Here's how the part is built. I have some questions about the finished solid (model axes, mm). Face numbers are marked on the shaded views. A direction names the side the tool comes from. Coordinates: 2 decimals unless noted, no trailing zeros. Write each loop counter-clockwise with the first axis right and the second up, starting at its lowest first coordinate (ties: lowest second). Pieces come first, ordered by that corner, then holes. Notation, with made-up numbers: (39, 11) - (49, 11) arc R21 ccw to (49, 34) - close; hole circle Ø7 at (29.25, 82). An arc over 180 degrees is marked (long way). Answer in a Markdown table with one row per item. Add a question column.
Item 1: If I drill on probe 1 along Y at (x, z) = (-159.65, 102.5); probe 2 along Z at (x, y) = (-158, 177); probe 3 along Y at (x, z) = (-159, -102), over which ranges is the centre line in solid material (lowest first)? Write a range as from..to.
Item 2: We'd pull the mould along Z, two halves only. Please class the marked faces 6, 7 and 8: +Z half, -Z half, draft (parallel to the pull), parting line (faces both ways), or undercut.
Item 3: Which directions (+Z, -Z, +X, -X, +Y, -Y) give clear straight access to the entire face, cutting with the end or side of a thin tool? Please do the marked faces 1, 2, 3, 4 and 5.
Item 4: Imagine slicing it at B-B (z = 41.5). Please give me the cut outline in (x, y).
Item 5: I'm going to push flat-ended pins straight in: pin 1 (6.5 mm diameter, centred on y = 6, z = -86, fed in from -X); pin 2 (1 mm diameter, centred on x = 98, y = 65, fed in from -Z); pin 3 (10 mm diameter, centred on x = -37, y = 99, fed in from +Z); pin 4 (1.5 mm diameter, centred on x = -83.5, z = 106.5, fed in from -Y). Where does each tip first touch, or does it pass through?
Item 6: Imagine slicing it at A-A (x = -112.5). Please give me the cut outline in (y, z).
from build123d import *

# Parameters (mm, degrees)
BOSS_EXTRUDE1_DEPTH = 170
SKETCH3_W           = 20
SKETCH3_H           = 25
SKETCH3_R           = 5
SKETCH3_W_2         = 30
SKETCH3_H_2         = 30
BOSS_EXTRUDE2_DEPTH = 5
FILLET1_R           = 5
SKETCH5_R           = 3
CUT_EXTRUDE1_DEPTH  = 3
BOSS_EXTRUDE5_DEPTH = 15
CHAMFER1_SIZE       = 5
FILLET2_R           = 5
SKETCH15_R          = 3
CUT_EXTRUDE2_DEPTH  = 5
SKETCH16_R          = 3
CUT_EXTRUDE3_DEPTH  = 5
SKETCH18_W          = 20
SKETCH18_H          = 165
CUT_EXTRUDE9_DEPTH  = 5
SKETCH21_W          = 20
SKETCH21_H          = 165
CUT_EXTRUDE10_DEPTH = 5


with BuildPart() as part:
    # Sketch1 → Boss-Extrude1 (new body)
    with BuildSketch(Plane(origin=(0, 0, 0), x_dir=(1, 0, 0), z_dir=(0, 1, 0))):
        Polygon((162.5, 80), (162.5, -80), (152.5, -80), (147.5, -80), (132.5, -80), (132.5, -95), (132.5, -100), (132.5, -110), (-102.5, -110), (-102.5, -100), (-102.5, -85), (-112.5, -85), (-122.5, -85), (-122.5, -100), (-122.5, -110), (-162.5, -110), (-162.5, -100), (-162.5, -95), (-132.5, -95), (-132.5, -85), (-132.5, -75), (-93.003639463, -75), (-93.003639463, -100), (122.5, -100), (122.5, -70), (152.5, -70), (152.5, 70), (122.5, 70), (122.5, 100), (-93.003639463, 100), (-93.003639463, 75), (-132.5, 75), (-132.5, 85), (-132.5, 95), (-162.5, 95), (-162.5, 100), (-162.5, 110), (-122.5, 110), (-122.5, 100), (-122.5, 85), (-112.5, 85), (-102.5, 85), (-102.5, 100), (-102.5, 110), (132.5, 110), (132.5, 100), (132.5, 95), (132.5, 80), (147.5, 80), (152.5, 80), align=None)
    extrude(amount=BOSS_EXTRUDE1_DEPTH)

    # Sketch3 → Boss-Extrude2 (add)
    # profile 1 of 4: a face of its own
    with BuildSketch(Plane(origin=(0, 0, 0), x_dir=(1, 0, 0), z_dir=(0, 1, 0))):
        with Locations((-112.5, -97.5)):
            Rectangle(SKETCH3_W, SKETCH3_H)
        with Locations(Location((-112.5, -95, 0), (0, 0, 270))):
            Circle(SKETCH3_R, mode=Mode.SUBTRACT)
    # profile 2 of 4: a face of its own
    with BuildSketch(Plane(origin=(0, 0, 0), x_dir=(1, 0, 0), z_dir=(0, 1, 0))):
        with Locations((147.5, -95)):
            Rectangle(SKETCH3_W_2, SKETCH3_H_2)
        with Locations(Location((147.5, -95, 0), (0, 0, 270))):
            Circle(SKETCH3_R, mode=Mode.SUBTRACT)
    # profile 3 of 4: a face of its own
    with BuildSketch(Plane(origin=(0, 0, 0), x_dir=(1, 0, 0), z_dir=(0, 1, 0))):
        with Locations((-112.5, 97.5)):
            Rectangle(SKETCH3_W, SKETCH3_H)
        with Locations(Location((-112.5, 95, 0), (0, 0, 90))):
            Circle(SKETCH3_R, mode=Mode.SUBTRACT)
    # profile 4 of 4: a face of its own
    with BuildSketch(Plane(origin=(0, 0, 0), x_dir=(1, 0, 0), z_dir=(0, 1, 0))):
        with Locations((147.5, 95)):
            Rectangle(SKETCH3_W_2, SKETCH3_H_2)
        with Locations(Location((147.5, 95, 0), (0, 0, 270))):
            Circle(SKETCH3_R, mode=Mode.SUBTRACT)
    extrude(amount=BOSS_EXTRUDE2_DEPTH)

    # Fillet1
    fillet1_edges = [part.edges().sort_by_distance(p)[0] for p in [
        (-122.5, 87.5, 85),
        (-102.5, 87.5, 85),
        (132.5, 87.5, 80),
        (132.5, 87.5, -80),
        (-102.5, 87.5, -85),
        (-122.5, 87.5, -85),
    ]]
    fillet(fillet1_edges, radius=FILLET1_R)

    # Sketch5 → Cut-Extrude1 (cut)
    with BuildSketch(Plane.ZY.offset(132.5)):
        with Locations((-85, 5)):
            Circle(SKETCH5_R)
        with Locations(Location((85, 5, 0), (0, 0, 180))):
            Circle(SKETCH5_R)
        with Locations((-85, 165)):
            Circle(SKETCH5_R)
        with Locations(Location((85, 165, 0), (0, 0, 180))):
            Circle(SKETCH5_R)
    extrude(amount=-CUT_EXTRUDE1_DEPTH, mode=Mode.SUBTRACT)

    # Sketch10 → Boss-Extrude5 (add)
    with BuildSketch(Plane(origin=(0, 170, 0), x_dir=(1, 0, 0), z_dir=(0, 1, 0))):
        Polygon((-162.5, 95), (-162.5, -95), (-162.5, -100), (-162.5, -110), (-122.5, -110), (-122.5, -100), (-122.5, -85), (-112.5, -85), (-102.5, -85), (-102.5, -100), (-102.5, -110), (132.5, -110), (132.5, -100), (132.5, -95), (132.5, -80), (147.5, -80), (152.5, -80), (162.5, -80), (162.5, 80), (152.5, 80), (147.5, 80), (132.5, 80), (132.5, 95), (132.5, 100), (132.5, 110), (-102.5, 110), (-102.5, 100), (-102.5, 85), (-112.5, 85), (-122.5, 85), (-122.5, 100), (-122.5, 110), (-162.5, 110), (-162.5, 100), align=None)
    extrude(amount=BOSS_EXTRUDE5_DEPTH)

    # Chamfer1
    chamfer1_edges = [part.edges().sort_by_distance(p)[0] for p in [
        (147.5, 185, -80),
        (15, 185, -110),
        (-142.5, 185, -110),
        (-142.5, 185, 110),
        (15, 185, 110),
        (147.5, 185, 80),
    ]]
    chamfer(chamfer1_edges, length=CHAMFER1_SIZE)

    # Fillet2
    fillet2_edges = [part.edges().sort_by_distance(p)[0] for p in [
        (-122.5, 177.5, -85),
        (-102.5, 177.5, -85),
        (132.5, 175, -80),
        (132.5, 175, 80),
        (-102.5, 177.5, 85),
        (-122.5, 177.5, 85),
    ]]
    fillet(fillet2_edges, radius=FILLET2_R)

    # Sketch15 → Cut-Extrude2 (cut)
    with BuildSketch(Plane.XZ):
        with Locations(Location((67.5, -105, 0), (0, 0, 90))):
            Circle(SKETCH15_R)
        with Locations(Location((-32.5, -105, 0), (0, 0, 90))):
            Circle(SKETCH15_R)
        with Locations(Location((157.5, -35, 0), (0, 0, 90))):
            Circle(SKETCH15_R)
        with Locations(Location((157.5, 35, 0), (0, 0, 270))):
            Circle(SKETCH15_R)
        with Locations(Location((67.5, 105, 0), (0, 0, 270))):
            Circle(SKETCH15_R)
        with Locations(Location((-32.5, 105, 0), (0, 0, 270))):
            Circle(SKETCH15_R)
    extrude(amount=-CUT_EXTRUDE2_DEPTH, mode=Mode.SUBTRACT)

    # Sketch16 → Cut-Extrude3 (cut)
    with BuildSketch(Plane.ZY.offset(162.5)):
        with Locations((-102.5, 177.5)):
            Circle(SKETCH16_R)
        with Locations((-102.5, 115.83)):
            Circle(SKETCH16_R)
        with Locations((-102.5, 54.16)):
            Circle(SKETCH16_R)
        with Locations((-34.17, 177.5)):
            Circle(SKETCH16_R)
        with Locations((34.16, 177.5)):
            Circle(SKETCH16_R)
        with Locations((102.49, 177.5)):
            Circle(SKETCH16_R)
        with Locations(Location((102.5, 54.16, 0), (0, 0, 180))):
            Circle(SKETCH16_R)
        with Locations(Location((102.5, 115.83, 0), (0, 0, 180))):
            Circle(SKETCH16_R)
    extrude(amount=-CUT_EXTRUDE3_DEPTH, mode=Mode.SUBTRACT)

    # Sketch18 → Cut-Extrude9 (cut)
    with BuildSketch(Plane.XY.offset(110)):
        with Locations((-35, 97.5)):
            Rectangle(SKETCH18_W, SKETCH18_H)
        with Locations((-10, 97.5)):
            Rectangle(SKETCH18_W, SKETCH18_H)
        with Locations((15, 97.5)):
            Rectangle(SKETCH18_W, SKETCH18_H)
        with Locations((40, 97.5)):
            Rectangle(SKETCH18_W, SKETCH18_H)
        with Locations((65, 97.5)):
            Rectangle(SKETCH18_W, SKETCH18_H)
        with Locations((90, 97.5)):
            Rectangle(SKETCH18_W, SKETCH18_H)
        with Locations((115, 97.5)):
            Rectangle(SKETCH18_W, SKETCH18_H)
        with Locations((-85, 97.5)):
            Rectangle(SKETCH18_W, SKETCH18_H)
        with Locations((-60, 97.5)):
            Rectangle(SKETCH18_W, SKETCH18_H)
    extrude(amount=-CUT_EXTRUDE9_DEPTH, mode=Mode.SUBTRACT)

    # Sketch21 → Cut-Extrude10 (cut)
    with BuildSketch(Plane(origin=(0, 0, -110), x_dir=(-1, 0, 0), z_dir=(0, 0, -1))):
        with Locations((-90, 97.5)):
            Rectangle(SKETCH21_W, SKETCH21_H)
        with Locations((-65, 97.5)):
            Rectangle(SKETCH21_W, SKETCH21_H)
        with Locations((-40, 97.5)):
            Rectangle(SKETCH21_W, SKETCH21_H)
        with Locations((-15, 97.5)):
            Rectangle(SKETCH21_W, SKETCH21_H)
        with Locations((10, 97.5)):
            Rectangle(SKETCH21_W, SKETCH21_H)
        with Locations((35, 97.5)):
            Rectangle(SKETCH21_W, SKETCH21_H)
        with Locations((60, 97.5)):
            Rectangle(SKETCH21_W, SKETCH21_H)
        with Locations((85, 97.5)):
            Rectangle(SKETCH21_W, SKETCH21_H)
        with Locations((-115, 97.5)):
            Rectangle(SKETCH21_W, SKETCH21_H)
    extrude(amount=-CUT_EXTRUDE10_DEPTH, mode=Mode.SUBTRACT)


solid = part.part
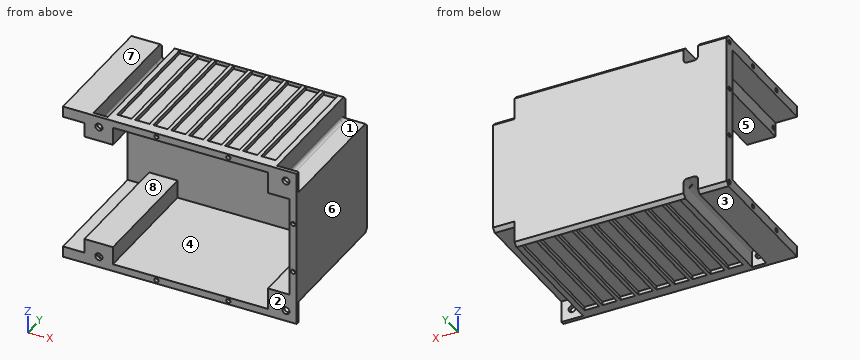
Here are the results:
| question | item | result |
|---|---|---|
| 1 | probe 1 | y = 0..51.16, 57.16..112.83, 118.83..174.5, 180.5..185 |
| 1 | probe 2 | z = -110..-105.46, -99.54..-37.13, -31.21..31.2, 37.12..99.53, 105.45..110 |
| 1 | probe 3 | y = 0..51.2, 57.12..112.87, 118.79..174.54, 180.46..185 |
| 2 | face 6 | draft |
| 2 | face 7 | +Z half |
| 2 | face 8 | undercut |
| 3 | face 1 | +Z, +X, +Y |
| 3 | face 2 | +Z, -Z, +X, -X, -Y |
| 3 | face 3 | -Z, +X, -X, +Y, -Y |
| 3 | face 4 | -Y |
| 3 | face 5 | -X, -Y |
| 4 | outline | (-162.5, 170) - (152.5, 170) - (152.5, 0) - (162.5, 0) - (162.5, 185) - (-162.5, 185) - close |
| 5 | pin 1 | stops at x = -132.5 |
| 5 | pin 2 | stops at z = -105 |
| 5 | pin 3 | stops at z = 105 |
| 5 | pin 4 | stops at y = 0 |
| 6 | outline | (0, -110) - (5, -110) - (5, -100) - (0, -100) - close; (0, -90) - (5, -90) - (5, -85) - (185, -85) - (185, 85) - (5, 85) - (5, 90) - (0, 90) - (0, 75) - (170, 75) - (170, -75) - (0, -75) - close; (0, 100) - (5, 100) - (5, 110) - (0, 110) - close |
